```python
from build123d import *

# Parameters (mm, degrees)
SKETCH1_W           = 69.85
SKETCH1_H           = 25.4
BOSS_EXTRUDE1_DEPTH = 3.175
FILLET1_R           = 6.35


with BuildPart() as part:
    # Sketch1 → Boss-Extrude1 (new body)
    with BuildSketch(Plane(origin=(0, 0, 0), x_dir=(1, 0, 0), z_dir=(0, 1, 0))):
        Polygon((254, 148.59), (254, 215.9), (0, 215.9), (0, 0), (254, 0), (254, 123.19), align=None)
        with Locations((212.725, 135.89)):
            Rectangle(SKETCH1_W, SKETCH1_H, mode=Mode.SUBTRACT)
    extrude(amount=BOSS_EXTRUDE1_DEPTH)

    # Fillet1
    fillet1_edges = [part.edges().sort_by_distance(p)[0] for p in [
        (0, 1.5875, -215.9),
        (254, 1.5875, -215.9),
        (254, 1.5875, 0),
        (0, 1.5875, 0),
        (177.8, 1.5875, -148.59),
        (177.8, 1.5875, -123.19),
        (247.65, 1.5875, -123.19),
        (247.65, 1.5875, -148.59),
    ]]
    fillet(fillet1_edges, radius=FILLET1_R)


solid = part.part
```
Build history of the part. All positions in model axes, mm. A direction names the side the tool comes from. Coordinates: 2 decimals unless noted, no trailing zeros. Order: outer loops, then holes, each group sorted by start corner. A loop starts at its lowest first (then second) coordinate and runs counter-clockwise, first axis right, second up. Notation, with made-up numbers: M 23,45 L 63,45 A16 ccw 63,57 Z; hole C 85,-9 d11. An arc over 180 degrees is marked long. One line per question, with ' | ' between items. Start each with the question number.
1. Wall check: line 1 along Z through (x, y) = (199.5, 2.4); line 2 along X through (y, z) = (1.9, -140.5); line 3 along X through (y, z) = (0.65, -124). Give the ranges that are in metal, low to high. Write a range as [from, to].
2. Mould opens along Z. For faces 1 (the face through (125, 0, -109)), 2 (the face through (179.71, 1.61, -146.78)), 3 (the face through (179.71, 1.61, -125)), 4 (the face through (1.81, 1.61, -1.91)) say: +Z half, -Z half, draft (parallel to the pull), parting line (faces both ways), or undercut.
3. Cut at B-B (y = 0.85). Write the cut outline in (x, z).
4. Cut at A-A (x = 212.5). Write the cut outline in (y, z) (3 decimals).
5. Tool access for faces 5 (the face through (252.19, 1.61, -1.91)), 6 (the face through (245.74, 1.61, -125)): list every direction of +Z, -Z, +X, -X, +Y, -Y with a clear straight run to the whole face (end or side of a thin tool).
The answers:
1) line 1: z = [-215.9, -148.59], [-123.19, 0] | line 2: x = [0, 177.8], [247.65, 254] | line 3: x = [0, 181.05], [244.4, 254]
2) face 1: draft | face 2: undercut | face 3: undercut | face 4: +Z half
3) outline: M 0,-209.55 A6.35 ccw 6.35,-215.9 L 247.65,-215.9 A6.35 ccw 254,-209.55 L 254,-6.35 A6.35 ccw 247.65,0 L 6.35,0 A6.35 ccw 0,-6.35 Z; hole M 177.8,-142.24 A6.35 ccw 184.15,-148.59 L 241.3,-148.59 A6.35 ccw 247.65,-142.24 L 247.65,-129.54 A6.35 ccw 241.3,-123.19 L 184.15,-123.19 A6.35 ccw 177.8,-129.54 Z
4) outline: M 0,-215.9 L 3.175,-215.9 L 3.175,-148.59 L 0,-148.59 Z; M 0,-123.19 L 3.175,-123.19 L 3.175,0 L 0,0 Z
5) face 5: +Z, +X, +Y, -Y | face 6: +Y, -Y
